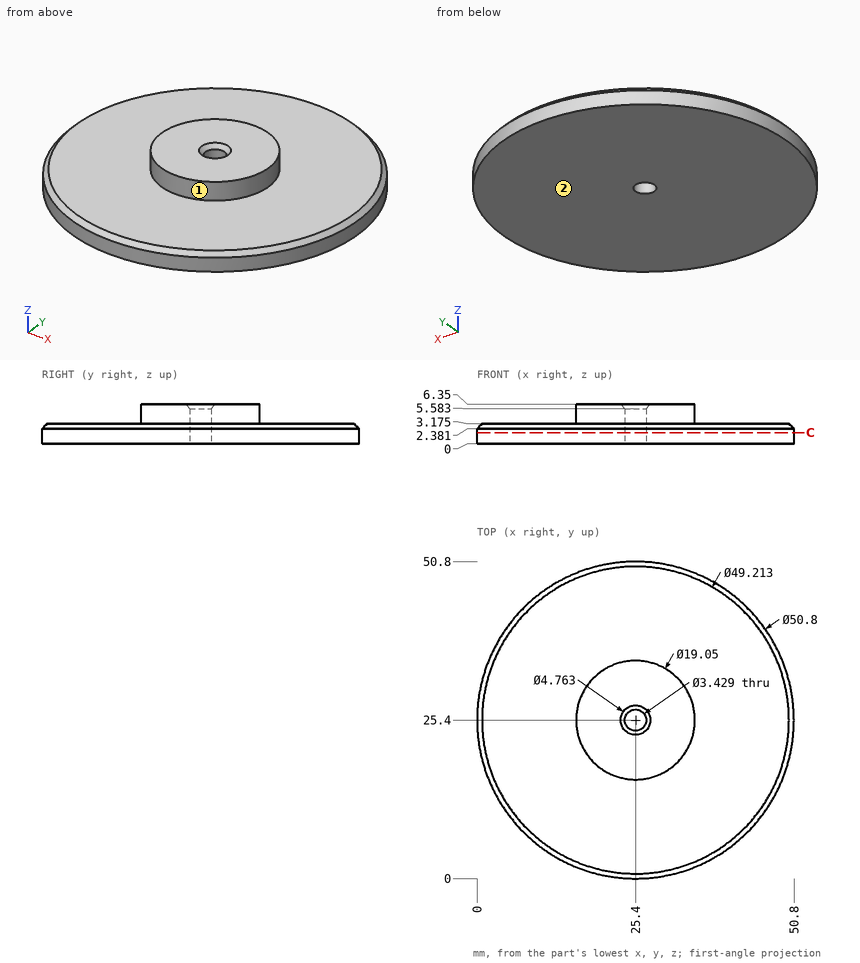
Check sheet for the drawn part. Datum: minimum x, y, z corner. Units: mm. A direction names the side the tool comes from. Give positions to 0.01 mm unless a question says otherwise; leave off trailing zeros. Order: outer loops, then holes, each group sorted by start corner. A loop starts at its lowest first (then second) coordinate and runs counter-clockwise, first axis right, second up. Notation, with made-up numbers: (-32, -22) -> (-18, -22) arc R24 cw to (-18, 13) -> close; hole circle Ø1 at (38, 50.25). An arc over 180 degrees is marked (long way). Use a Markdown table: item, result.
1) Material ranges on probe 1 along Y at (x, z) = (25.4, 2.1) (1 decimal); probe 2 along Y at (x, z) = (25.4, 4.35) (1 decimal); probe 3 along Z at (x, y) = (5, 33.5) (1 decimal), recorded low to high.
Results:
| item | result |
|---|---|
| probe 1 | 0 to 23.7, 27.1 to 50.8 |
| probe 2 | 15.9 to 23.7, 27.1 to 34.9 |
| probe 3 | 0 to 3.2 |
2) Tool access check on the marked faces 1 and 2. Record the directions out of +Z, -Z, +X, -X, +Y, -Y that give a thin tool (end or side, any length) a straight path to the whole face; none if there is none.
Results:
| item | result |
|---|---|
| face 1 | +Z |
| face 2 | -Z, +X, -X, +Y, -Y |
3) Depth check by flat-ended pin: pin 1 Ø15 at (x, y) = (16, 19) entering from +Z; pin 2 Ø1.5 at (x, z) = (11.5, 5) entering from -Y; pin 3 Ø4 at (x, y) = (22.5, 11.5) entering from +Z (1 decimal); pin 4 Ø2 at (x, z) = (10.5, 2) entering from -Y. Enter the tip coordinate at first touch or a pass-through.
Results:
| item | result |
|---|---|
| pin 1 | z = 6.35 |
| pin 2 | through |
| pin 3 | z = 3.2 |
| pin 4 | y = 4.14 |
4) Section check C-C, the plane z = 1.75. Record the boundary of the cut face in (x, y) (1 decimal).
Results:
| item | result |
|---|---|
| outline | circle Ø50.8 at (25.4, 25.4); hole circle Ø3.4 at (25.4, 25.4) |
